```python
from build123d import *

# Parameters (mm, degrees)
SKETCH1_R           = 4.9
SKETCH1_R_2         = 3.9
BOSS_EXTRUDE1_DEPTH = 10
CUT_EXTRUDE1_DEPTH  = 10


with BuildPart() as part:
    # Sketch1 → Boss-Extrude1 (new body)
    with BuildSketch(Plane.XY):
        Circle(SKETCH1_R)
        Circle(SKETCH1_R_2, mode=Mode.SUBTRACT)
    extrude(amount=BOSS_EXTRUDE1_DEPTH)

    # Sketch3 → Cut-Extrude1 (cut)
    with BuildSketch(Plane(origin=(4.9, 0, 0), x_dir=(0, 0, -1), z_dir=(1, 0, 0))):
        with BuildLine():
            Line((-10, 3.5), (-10, -3.5))
            Line((-10, -3.5), (-6, -3.5))
            ThreePointArc((-6, -3.5), (-4.570714214, 0), (-6, 3.5))
            Line((-6, 3.5), (-10, 3.5))
        make_face()
    extrude(amount=-CUT_EXTRUDE1_DEPTH, mode=Mode.SUBTRACT)


solid = part.part
```
Verification items for the finished model (mm, model axes). A direction names the side the tool comes from. Coordinates: 2 decimals unless noted, no trailing zeros. Write each loop counter-clockwise with the first axis right and the second up, starting at its lowest first coordinate (ties: lowest second). Pieces come first, ordered by that corner, then holes. Notation, with made-up numbers: (55, 26.25) - (112, 26.25) arc R19 ccw to (112, 41.25) - close; hole circle Ø11 at (33, 72.25). An arc over 180 degrees is marked (long way). One line per question, with ' | ' between items. Start each with the question number.
1. Section check D-D (x = 2). Enter the section's corners in (y, z).
2. Section check B-B (y = 0). Enter the section's corners in (x, z), plus the area to 3 significant figures.
3. Draft check along X on faces 3 (the flat face through (3, 3.5, 8)), 4 (the cylindrical face through (4.526, -1.877, 3.819)), 5 (the cylindrical face through (-3.896, 0.171, 3.819)). Enter one of: released by +X, released by -X, zero draft, split by the parting line, or undercut.
4. Gauge pin test, flat ends, axial feed: P1, Ø2, axis at x = -1, y = 2.5, coming from the +Z side; P2, Ø0.9, axis at x = 2.5, z = 9, coming from the +Y side; P3, Ø0.9, axis at x = -2.5, z = 7.5, coming from the -Y side; P4, Ø1.4, axis at x = 2.5, z = 8, coming from the -Y side. Record the tip position at first contact, or that the pin passes through.
5. Material ranges on line 1 along Y through (x, z) = (3.5, 2.5); line 2 along Y through (x, z) = (0, 3.25); line 3 along X through (y, z) = (-3, 3), recorded low to high.
6. Section check A-A (x = 0). Enter the section's corners in (y, z).
7. Access from +Z, -Z, +X, -X, +Y, -Y to the whole of each face (thin tool, end or side, straight path). Record for faces 1 (the flat face through (3, -3.5, 8)), 2 (the flat face through (0, 4.2, 10)).
8. Section check C-C (z = 3). Enter the section's corners in (x, y).
Computed values:
1) outline: (-4.47, 0) - (-3.35, 0) - (-3.35, 5.86) arc R5 cw to (-3.5, 6) - (-3.5, 10) - (-4.47, 10) - close; (3.35, 0) - (4.47, 0) - (4.47, 10) - (3.5, 10) - (3.5, 6) arc R5 cw to (3.35, 5.86) - close
2) outline: (-4.9, 0) - (-3.9, 0) - (-3.9, 4.57) - (-4.9, 4.57) - close; (3.9, 0) - (4.9, 0) - (4.9, 4.57) - (3.9, 4.57) - close | area: 9.14 mm²
3) face 3: zero draft | face 4: split by the parting line | face 5: undercut
4) P1: through | P2: y = 4.45 | P3: y = -4.45 | P4: y = -4.56
5) line 1: -3.43 to -1.72, 1.72 to 3.43 | line 2: -4.9 to -3.9, 3.9 to 4.9 | line 3: -3.87 to -2.49, 2.49 to 3.87
6) outline: (-4.9, 0) - (-3.9, 0) - (-3.9, 10) - (-4.9, 10) - close; (3.9, 0) - (4.9, 0) - (4.9, 10) - (3.9, 10) - close
7) face 1: +Z, +X, -X | face 2: +Z, +X, -X, +Y, -Y
8) outline: circle Ø9.8 at (0, 0); hole circle Ø7.8 at (0, 0)
